Verification items for the finished model (mm, model axes). Give positions to 0.01 mm unless a question says otherwise; leave off trailing zeros. Write each loop counter-clockwise with the first axis right and the second up, starting at its lowest first coordinate (ties: lowest second). Pieces come first, ordered by that corner, then holes. Notation, with made-up numbers: (85.25, 17.5) -> (109.25, 17.5) arc R22 ccw to (109.25, 41.5) -> close; hole circle Ø9 at (-32.5, -18.5). An arc over 180 degrees is marked (long way). Answer as CSV lines item,"result".
```python
from build123d import *

# Parameters (mm, degrees)
SKETCH003_R     = 8
PAD003_DEPTH    = 40
SKETCH004_R     = 1.5
POCKET_DEPTH    = 5
SKETCH005_R     = 7.45
POCKET001_DEPTH = 40.001


with BuildPart() as part:
    # Sketch003 → Pad003 (new body)
    with BuildSketch(Plane.XZ):
        with Locations((0, 15)):
            Circle(SKETCH003_R)
    extrude(amount=-PAD003_DEPTH)

    # Sketch004 (on DatumPlane) → Pocket (cut)
    with BuildSketch(Plane.XY.offset(10)):
        with Locations((0, 5)):
            Circle(SKETCH004_R)
    extrude(amount=-POCKET_DEPTH, mode=Mode.SUBTRACT)

    # Sketch005 → Pocket001 (cut, through all)
    with BuildSketch(Plane.XZ):
        with Locations((0, 15)):
            Circle(SKETCH005_R)
    extrude(amount=-POCKET001_DEPTH, mode=Mode.SUBTRACT)


with BuildPart() as part_1:
    # Body003 placement: moved
    add(part.part.moved(Location((0, -13, 0))))


solid = part_1.part
```
1) Section check A-A (z = 15). Record the boundary of the cut face in (x, y), and give its area (3 significant figures).
Reported:
outline,"(-8, -13) -> (-7.45, -13) -> (-7.45, 27) -> (-8, 27) -> close; (7.45, -13) -> (8, -13) -> (8, 27) -> (7.45, 27) -> close"
area,"44.0 mm²"
2) Draft check along X on faces 1 (the cylindrical face through (-1.73, 6.72, 7.19)), 2 (the cylindrical face through (-1.62, 6.72, 7.73)). Enter one of: +X half, -X half, draft (parallel to the pull), parting line (faces both ways), or undercut.
Reported:
face 1,"parting line"
face 2,"undercut"
3) Section check C-C (x = 4.25). Record the boundary of the cut face in (y, z), and give its area (3 significant figures).
Reported:
outline,"(-13, 8.22) -> (27, 8.22) -> (27, 8.88) -> (-13, 8.88) -> close; (-13, 21.12) -> (27, 21.12) -> (27, 21.78) -> (-13, 21.78) -> close"
area,"52.7 mm²"
4) Depth check by flat-ended pin: pin 1 (1.5 mm diameter, centred on y = -0.5, z = 12, fed in from +X); pin 2 (3.5 mm diameter, centred on x = 0, y = -8, fed in from -Z); pin 3 (4 mm diameter, centred on y = -4, z = 10, fed in from -X); pin 4 (3 mm diameter, centred on x = 3, y = 8.5, fed in from +Z). Enter the tip coordinate at first touch or a pass-through.
Reported:
pin 1,"x = 7.68"
pin 2,"z = 7"
pin 3,"x = -7.42"
pin 4,"z = 22.86"
5) Section check B-B (x = 0). Record the boundary of the cut face in (y, z).
Reported:
outline,"(-13, 7) -> (-9.5, 7) -> (-9.5, 7.55) -> (-13, 7.55) -> close; (-13, 22.45) -> (27, 22.45) -> (27, 23) -> (-13, 23) -> close; (-6.5, 7) -> (27, 7) -> (27, 7.55) -> (-6.5, 7.55) -> close"
6) Scan lines: line 1 along Y through (x, z) = (0, 7.4); line 2 along Z through (x, y) = (0, 7); line 3 along X through (y, z) = (12.5, 9.25). Record each from-to range of solid material in increasing order.
Reported:
line 1,"-13 to -9.5, -6.5 to 27"
line 2,"7 to 7.55, 22.45 to 23"
line 3,"-5.56 to -4.74, 4.74 to 5.56"
7) Section check D-D (y = 15). Record the boundary of the cut face in (x, z).
Reported:
outline,"circle Ø16 at (0, 15); hole circle Ø14.9 at (0, 15)"
